The listing builds one solid part. Answer for the finished solid, in the listing's coordinates (mm). A direction names the side the tool comes from. Round coordinates to 2 decimals unless told otherwise and drop trailing zeros. Order: outer loops, then holes, each group sorted by start corner. A loop starts at its lowest first (then second) coordinate and runs counter-clockwise, first axis right, second up. Notation, with made-up numbers: (13.5, -12) -> (24.5, -12) arc R10 ccw to (24.5, -5) -> close; hole circle Ø9 at (57, -38). An arc over 180 degrees is marked (long way). Return JSON: item names as keys, results as strings. Group by question number.
(1) The part is cut by section B-B (x = 0). Determine the outline of the cut face in (y, z).
(2) The part is cut by section D-D (z = 6). Determine the outline of the cut face in (x, y).
(3) Consider line 1 (X direction, y = 0, z = -27.25); line 2 (Y direction, x = 0, z = 29.75); line 3 (X direction, y = -0.25, z = -2.75). Determine where each line is inside the solid, lowest interval first. Write a range as [from, to].
(4) The part is cut by section A-A (z = -9.5). Determine the outline of the cut face in (x, y), plus the area to 3 significant figures.
(5) Which of the six approach directions +Z, -Z, +X, -X, +Y, -Y give full straight-line access (tool end or side, diameter ignored) to faces 1 (the face through (0, -2, 31)), 2 (the face through (0, -3, 36)), 3 (the face through (0, -1.25, -4))?
(6) Determine the mould class of faces 4 (the face through (0, -2, -8)), 5 (the face through (-6.2, -9.3, -36)) for opening direction X: +X half, -X half, draft (parallel to the pull), parting line (faces both ways), or undercut.
(7) Each of these flat-tipped pins is pushed along its axis until it touches: pin 1 (1 mm diameter, centred on x = 10.5, y = 11, fed in from +Z); pin 2 (11 mm diameter, centred on x = -4, y = 2, fed in from -Z); pin 3 (5 mm diameter, centred on y = -3.5, z = -10, fed in from +X); pin 4 (4 mm diameter, centred on x = 0, y = -0.25, fed in from +Z). Where does it stop, or does it pass through?
(8) The part is cut by section C-C (y = 10.25). Determine the outline of the cut face in (x, z).
Autodesk Inventor part; units mm, degrees
ref_plane "YZ Plane" through (0, 0, 0) normal (1, 0, 0) x (0, 1, 0)
ref_plane "XZ Plane" through (0, 0, 0) normal (0, 1, 0) x (-1, 0, 0)
ref_plane "XY Plane" through (0, 0, 0) normal (0, 0, 1) x (1, 0, 0)
sketch "Sketch1" plane through (0, 0, 0) normal (0, 0, 1) x (1, 0, 0)
  line L0 (-1.118, -1.25) -> (1.118, -1.25)
  arc A0 (1.118, -1.25) -> (-1.118, -1.25) centre (0, -0.25) ccw
  circle A1 centre (-0.0155, -0.3768) radius 13
  line L1 (7.9845, 2.6232) -> (7.9845, -0.3768)
  arc A2 (3.9845, -7.3768) -> (7.9845, -3.3768) centre (3.9845, -3.3768) ccw
  line L2 (3.9845, -7.3768) -> (-4.0155, -7.3768)
  arc A3 (-8.0155, -3.3768) -> (-4.0155, -7.3768) centre (-4.0155, -3.3768) ccw
  line L3 (-8.0155, -3.3768) -> (-8.0155, 2.6232)
  arc A4 (-6.0155, 6.0873) -> (-8.0155, 2.6232) centre (-4.0155, 2.6232) ccw
  line L4 (-6.0155, 6.0873) -> (-6.0155, -0.3768)
  arc A5 (-6.0155, -0.3768) -> (-3.3321, -5.3768) centre (-0.0155, -0.3768) ccw
  line L5 (-3.3321, -5.3768) -> (3.3011, -5.3768)
  arc A6 (3.3011, -5.3768) -> (5.9845, -0.3768) centre (-0.0155, -0.3768) ccw
  line L6 (5.9845, -0.3768) -> (5.9845, 6.0873)
  arc A7 (7.9845, 2.6232) -> (5.9845, 6.0873) centre (3.9845, 2.6232) ccw
  circle A8 centre (0, 0) radius 11
  line L7 (0, 11) -> (0, 14)
  circle A9 centre (0, 0) radius 14
  circle A10 centre (9.4845, -0.3768) radius 1.5
  line L8 (7.9845, -0.3768) -> (7.9845, -3.3768)
  dimension "d0" = 22
  dimension "d1" = 3
extrude "Extrusion1" add sketch "Sketch1" against normal blind 8 contours A8 | A1 | A9 | A10 | L1 L8 A2 L2 A3 L3 A4 L4 A5 L5 A6 L6 A7
sketch "Sketch2" plane through (0, 0, -8) normal (0, 0, -1) x (-1, 0, 0)
  circle A0 centre (0, 0) radius 14
  arc A1 (1.118, -1.25) -> (-1.118, -1.25) centre (0, -0.25) ccw
  line L0 (1.118, -1.25) -> (-1.118, -1.25)
  circle A2 centre (0, 0) radius 14
  line L1 (-14, 0) -> (-11, 0)
  circle A3 centre (0, 0) radius 11
  dimension "d4" = 3
extrude "Extrusion2" add sketch "Sketch2" along normal blind 28 contours A0
sketch "Sketch3" plane through (0, 0, 0) normal (0, 0, 1) x (1, 0, 0)
  circle A0 centre (0, 0) radius 14
extrude "Extrusion3" add sketch "Sketch3" along normal blind 36
sketch "Sketch4" plane through (0, 0, 36) normal (0, 0, 1) x (1, 0, 0)
  circle A0 centre (0, 0) radius 2
  point P0 (0, 0)
extrude "Extrusion4" cut sketch "Sketch4" against normal blind 10
properties material "Silicon Nitride"
Answer below:
{
 "1": {"outline": "(-14, -36) -> (-11, -36) -> (-11, -8) -> (-1.25, -8) -> (-1.25, 0) -> (1.25, 0) -> (1.25, -8) -> (11, -8) -> (11, -36) -> (14, -36) -> (14, 36) -> (2, 36) -> (2, 26) -> (-2, 26) -> (-2, 36) -> (-14, 36) -> close"},
 "2": {"outline": "circle Ø28 at (0, 0)"},
 "3": {"line 1": "x = [-14, -11], [11, 14]", "line 2": "y = [-14, -2], [2, 14]", "line 3": "x = [-14, -1.5], [1.5, 14]"},
 "4": {"outline": "circle Ø28 at (0, 0); hole circle Ø22 at (0, 0)", "area": "236 mm²"},
 "5": {"face 1": "+Z", "face 2": "+Z, +X, -X, +Y, -Y", "face 3": "-Z"},
 "6": {"face 4": "undercut", "face 5": "draft"},
 "7": {"pin 1": "passes through", "pin 2": "stops at z = -8", "pin 3": "stops at x = 13.96", "pin 4": "stops at z = 36"},
 "8": {"outline": "(-9.54, -36) -> (-3.99, -36) -> (-3.99, -8) -> (3.99, -8) -> (3.99, -36) -> (9.54, -36) -> (9.54, 36) -> (-9.54, 36) -> close"}
}
